The listing builds one solid part. Answer for the finished solid, in the listing's coordinates (mm). A direction names the side the tool comes from. Give positions to 0.01 mm unless a question says otherwise; leave off trailing zeros. Loops run counter-clockwise (first coordinate to the right, second up) from the corner with the lowest first, then second, coordinate; pieces in that order, holes last. Notation, with made-up numbers: M -28.75,-26.5 L 26.25,-26.5 A14 cw 26.25,-0.5 Z; hole C 63,-14 d4. An arc over 180 degrees is marked long. One line per item, written item: value. Start each with the question number.
Q1. A cutting plane is placed at B-B, the plane z = 5.5. Determine the outline of the cut face in (x, y), and give its area (3 significant figures).
Q2. A cutting plane is placed at D-D, the plane y = -6. Determine the outline of the cut face in (x, z), and give its area (3 significant figures).
Q3. A cutting plane is placed at C-C, the plane x = 5.5. Determine the outline of the cut face in (y, z).
Q4. The mould has two halves that part along X. Classify faces 5 (the flat face through (6.25, -12, 3)), 6 (the flat face through (-4.25, 2, 3)), 7 (the flat face through (0, 11, -1)): +X half, -X half, draft (parallel to the pull), parting line (faces both ways), or undercut.
Q5. Flat-ended cylindrical pins translate along their axes: pin 1 (1.5 mm diameter, centred on x = -7.5, z = 2.5, fed in from -Y); pin 2 (5.5 mm diameter, centred on x = 15, y = -1, fed in from -Z); pin 3 (1.5 mm diameter, centred on y = -11.5, z = 2, fed in from -X). Find the tip coordinate at first contact, or state that the pin passes through.
Q6. A cutting plane is placed at A-A, the plane y = 5.75. Determine the outline of the cut face in (x, z), and give its area (3 significant figures).
Q7. Consider L1, parallel to Y at x = 2.5, z = 5.5; L2, parallel to Z at x = -21, y = 0; L3, parallel to X at y = 4, z = 5.75. Determine where each line is inside the solid, lowest interval first.
Q8. For faces 1 (the flat face through (15, -10, 3)), 2 (the flat face through (-5, 3, 0.7)), 3 (the flat face through (-16, -10, 3)), 4 (the flat face through (15, 10, 3)), determine the directions among +Z, -Z, +X, -X, +Y, -Y from which every point of the face is accessible in a straight line to the end or side of a thin tool.
from build123d import *

# Parameters (mm, degrees)
F0_W      = 50
F0_H      = 20
F1_DEPTH  = 6
F2_W      = 12.5
F2_H      = 29.9
F3_DEPTH  = 6
F5_W      = 12.5
F5_H      = 21.55
F6_DEPTH  = 0.5
F8_W      = 3.5
F8_H      = 8
F9_DEPTH  = 0.2
F11_DEPTH = 1
F12_W     = 8.5
F12_H     = 6
F13_DEPTH = 25
F14_R     = 0.5


with BuildPart() as f1:
    # F0 (on Top) → F1 (new body)
    with BuildSketch(Plane.XY):
        Rectangle(F0_W, F0_H)
    extrude(amount=F1_DEPTH)

    # F2 (on face) → F3 (join)
    with BuildSketch(Plane(origin=(0, 0, 0), x_dir=(1, 0, 0), z_dir=(0, 0, -1))):
        Rectangle(F2_W, F2_H)
    extrude(amount=-F3_DEPTH)

    # F5 (on face) → F6 (cut)
    with BuildSketch(Plane(origin=(0, 0, 0), x_dir=(1, 0, 0), z_dir=(0, 0, -1))):
        with Locations((0, 4.175)):
            Rectangle(F5_W, F5_H)
    extrude(amount=-F6_DEPTH, mode=Mode.SUBTRACT)

    # F8 (on face) → F9 (cut)
    with BuildSketch(Plane(origin=(0, 0, 0.5), x_dir=(1, 0, 0), z_dir=(0, 0, -1))):
        with Locations((-4.5, -2.6)):
            Rectangle(F8_W, F8_H)
    extrude(amount=-F9_DEPTH, mode=Mode.SUBTRACT)

    # F10 (on face) → F11 (join)
    with BuildSketch(Plane(origin=(0, 0, 0), x_dir=(1, 0, 0), z_dir=(0, 0, -1))):
        Polygon((-6.25, -10), (-6.25, -14.95), (6.25, -14.95), (6.25, -6.6), (-6.25, -6.6), align=None)
    extrude(amount=F11_DEPTH)

    # F12 (on face) → F13 (cut)
    with BuildSketch(Plane(origin=(0, 0, 0.5), x_dir=(1, 0, 0), z_dir=(0, 0, -1))):
        with Locations((0, -1.6)):
            Rectangle(F12_W, F12_H)
    extrude(amount=-F13_DEPTH, mode=Mode.SUBTRACT)

    # F14
    f14_edges = [f1.edges().sort_by_distance(p)[0] for p in [
        (4.25, -1.4, 3.25),
        (4.25, 4.6, 3.25),
        (-4.25, 4.6, 3.35),
        (-4.25, -1.4, 3.35),
    ]]
    fillet(f14_edges, radius=F14_R)


solid = f1.part
Answer block:
1. outline: M -25,-10 L -6.25,-10 L -6.25,-14.95 L 6.25,-14.95 L 6.25,-10 L 25,-10 L 25,10 L 6.25,10 L 6.25,14.95 L -6.25,14.95 L -6.25,10 L -25,10 Z; hole M -4.25,-0.9 A0.5 ccw -3.75,-1.4 L 3.75,-1.4 A0.5 ccw 4.25,-0.9 L 4.25,4.1 A0.5 ccw 3.75,4.6 L -3.75,4.6 A0.5 ccw -4.25,4.1 Z
1. area: 1,070 mm^2
2. outline: M -25,0 L -6.25,0 L -6.25,0.5 L 6.25,0.5 L 6.25,0 L 25,0 L 25,6 L -25,6 Z
2. area: 294 mm^2
3. outline: M -14.95,0.5 L 6.6,0.5 L 6.6,-1 L 14.95,-1 L 14.95,6 L -14.95,6 Z
4. face 5: +X half
4. face 6: undercut
4. face 7: draft
5. pin 1: y = -10
5. pin 2: z = 0
5. pin 3: x = -6.25
6. outline: M -25,0 L -6.25,0 L -6.25,0.7 L -2.75,0.7 L -2.75,0.5 L 6.25,0.5 L 6.25,0 L 25,0 L 25,6 L -25,6 Z
6. area: 293 mm^2
7. L1: -14.95 to -1.4, 4.6 to 14.95
7. L2: 0 to 6
7. L3: -25 to -4.25, 4.25 to 25
8. face 1: +Z, -Z, +X, -Y
8. face 2: -Z
8. face 3: +Z, -Z, -X, -Y
8. face 4: +Z, -Z, +X, +Y
